Source: CAD feature listing. Evaluate the final solid. Frame: model axes, mm. Face numbers are marked on the shaded views. A direction names the side the tool comes from. Round coordinates to 2 decimals unless told otherwise and drop trailing zeros. Write each loop counter-clockwise with the first axis right and the second up, starting at its lowest first coordinate (ties: lowest second). Pieces come first, ordered by that corner, then holes. Notation, with made-up numbers: (35.25, 5.25) -> (51.25, 5.25) arc R15 ccw to (51.25, 19.25) -> close; hole circle Ø3 at (58.5, -35). An arc over 180 degrees is marked (long way). Put each result on its own line as item: value.
```python
from build123d import *

# Parameters (mm, degrees)
SKETCH1_R               = 10
BOSS_EXTRUDE1_DEPTH     = 65
BOSS_EXTRUDE2_DEPTH     = 10
BOSS_EXTRUDE3_DEPTH     = 65
SKETCH4_R               = 4.05
CUT_EXTRUDE1_DEPTH      = 84.964278119
FILLET1_R               = 10
FILLET2_R               = 2
CUT_EXTRUDE2_DEPTH      = 90.162772501
CUT_EXTRUDE2_DEPTH_BACK = 90.162772501
SKETCH6_R               = 4.05
SKETCH7_W               = 12
SKETCH7_H               = 35
CUT_EXTRUDE3_DEPTH      = 90.162772501
BOSS_EXTRUDE4_REACH     = 88.637
SKETCH8_R               = 4


with BuildPart() as part:
    # Sketch1 → Boss-Extrude1 (new body)
    with BuildSketch(Plane(origin=(0, 0, 0), x_dir=(1, 0, 0), z_dir=(0, 1, 0))):
        with Locations(Location((0, 0, 0), (0, 0, 270))):
            Circle(SKETCH1_R)
    extrude(amount=-BOSS_EXTRUDE1_DEPTH)

    # Sketch2 → Boss-Extrude2 (add)
    with BuildSketch(Plane(origin=(0, 0, 0), x_dir=(1, 0, 0), z_dir=(0, 1, 0))):
        with BuildLine():
            Line((0, -10), (35, -10))
            Line((35, -10), (35, 40))
            Line((35, 40), (-10, 40))
            Line((-10, 40), (-10, 0))
            ThreePointArc((-10, 0), (-7.071067812, -7.071067812), (0, -10))
        make_face()
    extrude(amount=-BOSS_EXTRUDE2_DEPTH)

    # Sketch3 → Boss-Extrude3 (add)
    with BuildSketch(Plane(origin=(0, 0, 0), x_dir=(1, 0, 0), z_dir=(0, 1, 0))):
        with BuildLine():
            Line((35, -10), (35, 40))
            Line((35, 40), (15, 40))
            Line((15, 40), (15, 10))
            Line((15, 10), (0, 10))
            ThreePointArc((0, 10), (-7.071067812, 7.071067812), (-10, 0))
            ThreePointArc((-10, 0), (-7.071067812, -7.071067812), (0, -10))
            Line((0, -10), (35, -10))
        make_face()
    extrude(amount=-BOSS_EXTRUDE3_DEPTH)

    # Sketch4 → Cut-Extrude1 (cut, through all)
    with BuildSketch(Plane(origin=(0, 0, 0), x_dir=(1, 0, 0), z_dir=(0, 1, 0))):
        with Locations(Location((0, 0, 0), (0, 0, 270))):
            Circle(SKETCH4_R)
        with Locations(Location((0, 31.15, 0), (0, 0, 270))):
            Circle(SKETCH4_R)
    extrude(amount=-CUT_EXTRUDE1_DEPTH, mode=Mode.SUBTRACT)

    # Fillet1
    fillet1_edges = [part.edges().sort_by_distance(p)[0] for p in [
        (-10, -5, -40),
    ]]
    fillet(fillet1_edges, radius=FILLET1_R)

    # Fillet2
    fillet2_edges = [part.edges().sort_by_distance(p)[0] for p in [
        (35, -32.5, 10),
        (17.5, 0, 10),
        (35, 0, -15),
        (17.5, 0, -40),
        (-10, -65, 0),
        (7.5, -65, -10),
        (15, -65, -25),
        (25, -65, -40),
        (35, -65, -15),
        (17.5, -65, 10),
        (-7.071067812, 0, 7.071067812),
        (-10, 0, -15),
        (-7.071067812, 0, -37.071067812),
        (35, -32.5, -40),
    ]]
    fillet(fillet2_edges, radius=FILLET2_R)

    # Sketch6 → Cut-Extrude2 (cut, two sides: drawn at the far end of the back side and taken through both)
    with BuildSketch(Plane(origin=(0, 0, -40), x_dir=(-1, 0, 0), z_dir=(0, 0, -1)).offset(-CUT_EXTRUDE2_DEPTH_BACK)):
        with Locations((-24.999085547, -7.5)):
            Circle(SKETCH6_R)
        with Locations((-24.999085547, -57.5)):
            Circle(SKETCH6_R)
    extrude(amount=CUT_EXTRUDE2_DEPTH + CUT_EXTRUDE2_DEPTH_BACK, mode=Mode.SUBTRACT)

    # Sketch7 → Cut-Extrude3 (cut, through all)
    with BuildSketch(Plane(origin=(0, 0, -40), x_dir=(-1, 0, 0), z_dir=(0, 0, -1))):
        with Locations((-25, -32.5)):
            Rectangle(SKETCH7_W, SKETCH7_H)
    extrude(amount=-CUT_EXTRUDE3_DEPTH, mode=Mode.SUBTRACT)

    # Sketch8 → Boss-Extrude4 (add, up to next)
    with BuildSketch(Plane.ZY.offset(-31), mode=Mode.PRIVATE) as boss_extrude4_sk1:
        with Locations(Location((0, -32.5, 0), (0, 0, 90))):
            Circle(SKETCH8_R)
    boss_extrude4_tool1 = extrude(boss_extrude4_sk1.sketch, amount=BOSS_EXTRUDE4_REACH, mode=Mode.PRIVATE) - part.part
    add(boss_extrude4_tool1.solids().sort_by_distance((31, -32.5, 0))[0])


solid = part.part
```
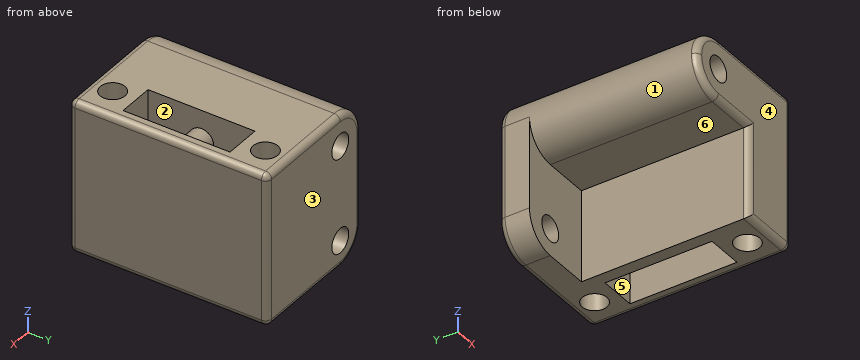
Q1. Draft query along X for the marked faces 1, 2 and 3. Return one class per face: +X half, -X half, draft (parallel to the pull), parting line (faces both ways), or undercut.
Ans:
face 1: -X half
face 2: undercut
face 3: draft
Q2. Pin query (flat end, axial travel): pin 1 (10.5 mm diameter, centred on y = -24, z = -8.5, fed in from -X); pin 2 (10 mm diameter, centred on x = -2, z = -30, fed in from -Y); pin 3 (4.5 mm diameter, centred on x = 9.5, y = -30, fed in from -Z). Return the tip coordinate at first contact, or that it passes through.
Ans:
pin 1: stops at x = -9.46
pin 2: stops at y = -10
pin 3: stops at z = -10
Q3. Cut plane C-C on y = -7.5. Output: boundary loops of the cut face in (x, z).
Ans:
outline: (-10, -30) arc R10 ccw to (0, -40) -> (20.95, -40) -> (20.95, 10) -> (0, 10) arc R10 ccw to (-10, 0) -> close; (29.05, -40) -> (33, -40) arc R2 ccw to (35, -38) -> (35, 8) arc R2 ccw to (33, 10) -> (29.05, 10) -> close; hole circle Ø8.1 at (0, -31.15); hole circle Ø8.1 at (0, 0)
Q4. Material intervals for line 1 (Y direction, x = 27.5, z = -8); line 2 (X direction, y = -7.5, z = -21); line 3 (X direction, y = -23.5, z = -18), sorted ascending. Write a range as [from, to].
Ans:
line 1: y = [-65, -60.69], [-54.31, -50], [-15, -10.69], [-4.31, 0]
line 2: x = [-10, 20.95], [29.05, 35]
line 3: x = [15, 19], [31, 35]
Q5. Cut plane D-D on x = 7. Output: boundary loops of the cut face in (y, z).
Ans:
outline: (-65, -8) arc R2 ccw to (-63, -10) -> (-10, -10) -> (-10, -40) -> (-2, -40) arc R2 ccw to (0, -38) -> (0, 8) arc R2 ccw to (-2, 10) -> (-63, 10) arc R2 ccw to (-65, 8) -> close
Q6. Cut plane B-B on z = -11. Output: boundary loops of the cut face in (x, y).
Ans:
outline: (-10, -10) -> (15, -10) -> (15, -63) arc R2 ccw to (17, -65) -> (33, -65) arc R2 ccw to (35, -63) -> (35, -2) arc R2 ccw to (33, 0) -> (-8, 0) arc R2 ccw to (-10, -2) -> close; hole (19, -50) -> (31, -50) -> (31, -15) -> (19, -15) -> close; hole circle Ø8.1 at (25, -57.5); hole circle Ø8.1 at (25, -7.5)
Q7. Reachability of the marked faces 4, 5 and 6 from +Z, -Z, +X, -X, +Y, -Y: full face, straight path, thin tool, end or side. Return the list, or none.
Ans:
face 4: +Z, -Z, +X, -X, -Y
face 5: +Z, -Z
face 6: -Z, -X, -Y
Q8. Cut plane A-A on y = -47. Output: boundary loops of the cut face in (x, z).
Ans:
outline: (0, -10) -> (15, -10) -> (15, -40) -> (19, -40) -> (19, 10) -> (0, 10) arc R10 ccw to start; (31, -40) -> (33, -40) arc R2 ccw to (35, -38) -> (35, 8) arc R2 ccw to (33, 10) -> (31, 10) -> close; hole circle Ø8.1 at (0, 0)
